```python
from build123d import *

# Parameters (mm, degrees)
F0_W     = 863.6
F0_H     = 914.4
F1_DEPTH = 228.6
F4_DEPTH = 457.201
F5_DEPTH = 863.601
F6_T     = -19.05


with BuildPart() as f1:
    # F0 (on Front) → F1 (new body, symmetric)
    with BuildSketch(Plane.XZ):
        Rectangle(F0_W, F0_H)
    extrude(amount=F1_DEPTH, both=True)

    # F2 (on face) → F4 (cut, through all)
    with BuildSketch(Plane.XZ.offset(228.6)):
        Polygon((-127, -457.2), (-431.8, 457.2), (-431.8, -457.2), align=None)
        Polygon((431.8, -457.2), (431.8, 457.2), (127, -457.2), align=None)
    extrude(amount=-F4_DEPTH, mode=Mode.SUBTRACT)

    # F3 (on face) → F5 (cut, through all)
    with BuildSketch(Plane(origin=(-431.8, 0, 0), x_dir=(0, -1, 0), z_dir=(-1, 0, 0))):
        Polygon((-76.2, -457.2), (-228.6, 457.2), (-228.6, -457.2), align=None)
        Polygon((228.6, -457.2), (228.6, 457.2), (76.2, -457.2), align=None)
    extrude(amount=-F5_DEPTH, mode=Mode.SUBTRACT)

    # F6
    f6_openings = [f1.faces().sort_by_distance(p)[0] for p in [
        (0, 0, 457.2),
    ]]
    offset(amount=F6_T, openings=f6_openings)


solid = f1.part
```
Part model, mm, in its own coordinate system. A direction names the side the tool comes from. Round coordinates to 2 decimals unless told otherwise and drop trailing zeros. Write each loop counter-clockwise with the first axis right and the second up, starting at its lowest first coordinate (ties: lowest second). Pieces come first, ordered by that corner, then holes. Notation, with made-up numbers: (56, 5.25) -> (77, 5.25) arc R19 cw to (77, 18.25) -> close; hole circle Ø10 at (41, -17). An arc over 180 degrees is marked (long way). Return JSON: item names as keys, results as strings. Group by question number.
Q1. Probe L1, parallel to Y at x = -179.5, z = 147; L2, parallel to X at y = -88, z = 331; L3, parallel to Y at x = 245, z = 172.5. List the from-to ranges inside material, lowest first. Write a range as [from, to].
Q2. Pin check, flat tips, straight feed: pin 1 (6 mm diameter, centred on y = 143, z = 76, fed in from -X); pin 2 (6 mm diameter, centred on x = 82.5, z = 235, fed in from -Y); pin 3 (8 mm diameter, centred on x = -109.5, z = -238, fed in from +Y). Stop position of each tip, or through.
Q3. Saw through at B-B on x = 82. Write the cut outline in (y, z).
Q4. Saw through at A-A on y = -1.5. Write the cut outline in (x, z), plus the area to 3 significant figures.
Q5. Which spindle directions (+Z, -Z, +X, -X, +Y, -Y) get a long thin tool onto all of the face, cutting with end or side? Do faces 1 (the flat face through (-2, -1, -438.15)), 2 (the flat face through (-311.133, -3.2, 95.199)). Say none if no direction does.
Q6. Saw through at C-C on z = -290. Write the cut outline in (x, y).
Q7. Saw through at D-D on z = 16. Write the cut outline in (x, y).
Q8. Mould opens along Y. For faces 3 (the flat face through (-6, -170.4, 108)), 4 (the flat face through (-6.045, 168.267, 95.199)), 5 (the flat face through (-5.76, 150.21, 102.74)), 6 (the flat face through (-2, -1, -457.2)) say: pulls with the +Y half, pulls with the -Y half, needs draft (parallel to the pull), parting line crosses it, or undercut.
Answer:
{
 "1": {"L1": "[-176.9, -157.59], [157.59, 176.9]", "L2": "[-389.73, -369.65], [369.65, 389.73]", "L3": "[-181.15, -161.84], [161.84, 181.15]"},
 "2": {"pin 1": "x = -305.73", "pin 2": "y = -192.07", "pin 3": "y = 113.4"},
 "3": {"outline": "(-228.6, 457.2) -> (-76.2, -457.2) -> (76.2, -457.2) -> (228.6, 457.2) -> (209.29, 457.2) -> (60.06, -438.15) -> (-60.06, -438.15) -> (-209.29, 457.2) -> close"},
 "4": {"outline": "(-431.8, 457.2) -> (-127, -457.2) -> (127, -457.2) -> (431.8, 457.2) -> (411.72, 457.2) -> (113.27, -438.15) -> (-113.27, -438.15) -> (-411.72, 457.2) -> close", "area": "40,900 mm2"},
 "5": {"face 1": "+Z", "face 2": "-Z, -X, +Y, -Y"},
 "6": {"outline": "(-182.73, -104.07) -> (182.73, -104.07) -> (182.73, 104.07) -> (-182.73, 104.07) -> close; hole (-162.65, -84.75) -> (162.65, -84.75) -> (162.65, 84.75) -> (-162.65, 84.75) -> close"},
 "7": {"outline": "(-284.73, -155.07) -> (284.73, -155.07) -> (284.73, 155.07) -> (-284.73, 155.07) -> close; hole (-264.65, -135.75) -> (264.65, -135.75) -> (264.65, 135.75) -> (-264.65, 135.75) -> close"},
 "8": {"face 3": "pulls with the -Y half", "face 4": "pulls with the +Y half", "face 5": "undercut", "face 6": "needs draft"}
}
